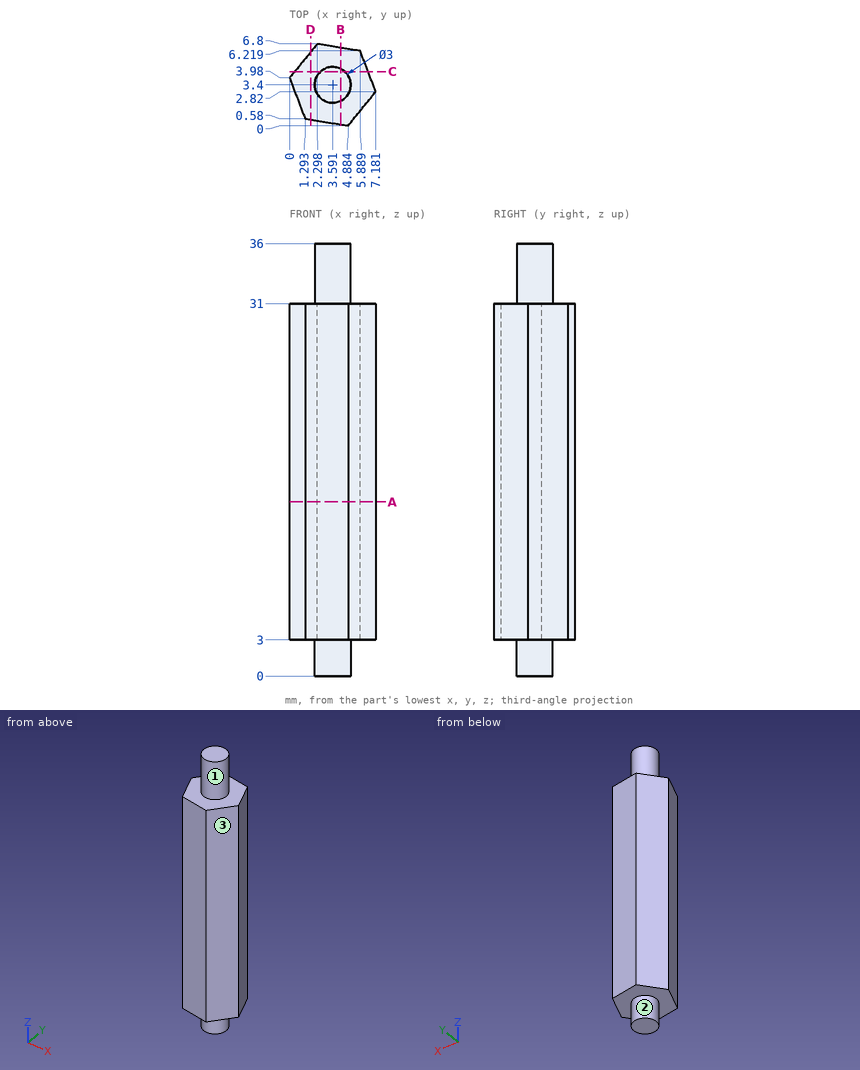
The drawing under review shows one solid part. Ordinate dimensions are in mm from its lowest x, y, z. A direction names the side the tool comes from. Give positions to 0.01 mm unless a question says otherwise; leave off trailing zeros. Order: outer loops, then holes, each group sorted by start corner. A loop starts at its lowest first (then second) coordinate and runs counter-clockwise, first axis right, second up. Notation, with made-up numbers: M -26.75,-24.75 L 20.25,-24.75 A24 ccw 20.25,-1.75 Z; hole C -12,85 d5. An arc over 180 degrees is marked long. One line per question, with ' | ' between items. Start each with the question number.
Q1. For L1, parallel to Z at x = 3.5, y = 5.5; L2, parallel to Y at x = 2.75, z = 30 (1 decimal); L3, parallel to X at y = 5, z = 11, list the stretches that pass through material, from the lowest coordinate up. Write a range as [from, to].
Q2. We need section C-C (y = 4.5). Write out the cut boundary in (x, z), plus the area to 3 significant figures.
Q3. We need section A-A (z = 14.5). Write out the cut boundary in (x, y).
Q4. We need section D-D (x = 1.75). Write out the cut boundary in (y, z).
Q5. For pin 1 Ø3 at (y, z) = (4, 21.5) entering from +X; pin 2 Ø1 at (x, z) = (1, 24) entering from +Y; pin 3 Ø1.5 at (y, z) = (1.5, 25.5) entering from +X, all flat-tipped, find the tip position at first contact; note any pin that passes through.
Q6. We need section B-B (x = 4.25). Write out the cut boundary in (y, z) (1 decimal).
Q7. Machinability: for the marked faces 1, 2 and 3, which of the approach directions +Z, -Z, +X, -X, +Y, -Y give a long, thin tool a straight path to every point of the face, cutting with its end or side? Answer none if there is none.
Returned:
1) L1: [3, 31] | L2: [0.3, 6.7] | L3: [0.83, 6.35]
2) outline: M 0.42,3 L 2.57,3 L 2.57,0 L 4.61,0 L 4.61,3 L 6.54,3 L 6.54,31 L 4.61,31 L 4.61,36 L 2.57,36 L 2.57,31 L 0.42,31 Z | area: 188 mm2
3) outline: M 0,3.98 L 1.29,0.58 L 4.88,0 L 7.18,2.82 L 5.89,6.22 L 2.3,6.8 Z
4) outline: M 0.51,3 L 6.13,3 L 6.13,31 L 0.51,31 Z
5) pin 1: x = 7.18 | pin 2: y = 5.82 | pin 3: x = 6.72
6) outline: M 0.1,3 L 2.1,3 L 2.1,0 L 4.7,0 L 4.7,3 L 6.5,3 L 6.5,31 L 4.7,31 L 4.7,36 L 2.1,36 L 2.1,31 L 0.1,31 Z
7) face 1: +Z | face 2: -Z | face 3: +Z, -Z, +X, -Y
